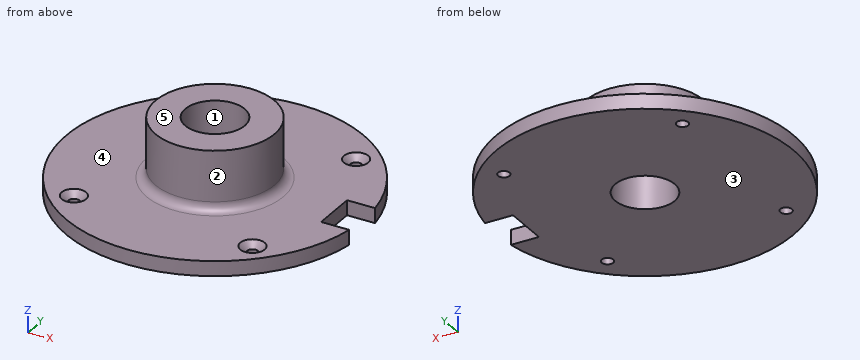
```python
from build123d import *

# Parameters (mm, degrees)
SKETCH5_W                                         = 10
SKETCH5_H                                         = 15
EXTRUDE2_DEPTH                                    = 6
CSK_FOR_M3_5_FLAT_HEAD_MACHINE_SCREW1_D           = 3.9
CSK_FOR_M3_5_FLAT_HEAD_MACHINE_SCREW1_CSINK_D     = 8.2
CSK_FOR_M3_5_FLAT_HEAD_MACHINE_SCREW1_CSINK_ANGLE = 90
CIRPATTERN1_COUNT                                 = 4


with BuildPart() as part:
    # Sketch1 → Revolve1 (revolve)
    with BuildSketch(Plane(origin=(0, 0, 0), x_dir=(0, 0, -1), z_dir=(1, 0, 0))):
        with BuildLine():
            Line((0, 10), (-25, 10))
            Line((-25, 10), (-25, 20))
            Line((-25, 20), (-8, 20))
            ThreePointArc((-8, 20), (-5.878679656, 20.878679656), (-5, 23))
            Line((-5, 23), (-5, 50))
            Line((-5, 50), (0, 50))
            Line((0, 50), (0, 10))
        make_face()
    revolve(axis=Axis((0, 0, 50), (0, 0, -1)))

    # Sketch5 → Extrude2 (cut, through all)
    with BuildSketch(Plane.XY.offset(5)):
        with Locations((45, 0)):
            Rectangle(SKETCH5_W, SKETCH5_H)
    extrude(amount=-EXTRUDE2_DEPTH, mode=Mode.SUBTRACT)

    # CSK for M3.5 Flat Head Machine Screw1 (through all)
    with Locations(Plane.XY.offset(5)):
        with Locations((-30, 30)):
            csk_for_m3_5_flat_head_machine_screw1 = CounterSinkHole(CSK_FOR_M3_5_FLAT_HEAD_MACHINE_SCREW1_D / 2, CSK_FOR_M3_5_FLAT_HEAD_MACHINE_SCREW1_CSINK_D / 2, counter_sink_angle=CSK_FOR_M3_5_FLAT_HEAD_MACHINE_SCREW1_CSINK_ANGLE)

    # CirPattern1: CSK for M3.5 Flat Head Machine Screw1 ×4 about axis
    cirpattern1_axis = Axis((0, 0, 0), (0, 0, 1))
    for i in range(1, CIRPATTERN1_COUNT):
        add(csk_for_m3_5_flat_head_machine_screw1.rotate(cirpattern1_axis, i * 360 / CIRPATTERN1_COUNT), mode=Mode.SUBTRACT)


solid = part.part
```
Can you work these out from the model? Positions are in its coordinate system, mm. Face numbers are marked on the shaded views. A direction names the side the tool comes from. Round coordinates to 2 decimals unless told otherwise and drop trailing zeros. Loops run counter-clockwise (first coordinate to the right, second up) from the corner with the lowest first, then second, coordinate; pieces in that order, holes last. Notation, with made-up numbers: (81, 5) -> (88, 5) arc R22 ccw to (88, 21) -> close; hole circle Ø9 at (40.25, -17). An arc over 180 degrees is marked (long way). One line per item, written item: value. Start each with the question number.
1. If we section it at D-D, the plane z = 21: Write out the boundary of the cut face in (x, y).
2. If I drill on probe 1 along X at (y, z) = (-30, 0.85); probe 2 along Z at (x, y) = (-22.5, -23); probe 3 along X at (y, z) = (3, 13), over which ranges is the centre line in solid material (lowest first)?
3. For pin 1 (2 mm diameter, centred on x = -12.5, z = 3, fed in from +Y); pin 2 (4 mm diameter, centred on x = 45.5, z = 1.5, fed in from +Y); pin 3 (6 mm diameter, centred on x = -35, z = 5.5, fed in from +Y), each with a flat end and sliding along its axis, tell me the tip position at first contact or that it passes through.
4. If we mould it in two halves opening along Y, with no side actions, what happens to the marked faces 1, 2 and 3? For each: pulls with the +Y half, pulls with the -Y half, needs draft (parallel to the pull), parting line crosses it, or undercut.
5. For the marked faces 4 and 5, which set-ups out of +Z, -Z, +X, -X, +Y, -Y let a thin tool reach every point of the face, with its end or its side?
6. If we section it at A-A, the plane x = -30: Write out the boundary of the cut face in (y, z).
7. If we section it at C-C, the plane x = 0: Write out the boundary of the cut face in (y, z), then the cut area to 3 significant figures.
Calculated:
1. outline: circle Ø40 at (0, 0); hole circle Ø20 at (0, 0)
2. probe 1: x = -40 to -31.95, -28.05 to 28.05, 31.95 to 40
2. probe 2: z = 0 to 5
2. probe 3: x = -19.77 to -9.54, 9.54 to 19.77
3. pin 1: stops at y = 48.66
3. pin 2: stops at y = 24.65
3. pin 3: stops at y = 38.38
4. face 1: undercut
4. face 2: parting line crosses it
4. face 3: needs draft
5. face 4: +Z
5. face 5: +Z, +X, -X, +Y, -Y
6. outline: (-40, 0) -> (-31.95, 0) -> (-31.95, 2.85) -> (-34.1, 5) -> (-40, 5) -> close; (-28.05, 0) -> (28.05, 0) -> (28.05, 2.85) -> (25.9, 5) -> (-25.9, 5) -> (-28.05, 2.85) -> close; (31.95, 0) -> (40, 0) -> (40, 5) -> (34.1, 5) -> (31.95, 2.85) -> close
7. outline: (-50, 0) -> (-10, 0) -> (-10, 25) -> (-20, 25) -> (-20, 8) arc R3 cw to (-23, 5) -> (-50, 5) -> close; (10, 0) -> (50, 0) -> (50, 5) -> (23, 5) arc R3 cw to (20, 8) -> (20, 25) -> (10, 25) -> close
7. area: 804 mm²
